Input: part model. Units: mm. Frame: model coordinates. Face numbers are marked on the shaded views. A direction names the side the tool comes from. Give positions to 0.01 mm unless a question says otherwise; leave off trailing zeros. Write each loop counter-clockwise with the first axis right and the second up, starting at its lowest first coordinate (ties: lowest second). Pieces come first, ordered by that corner, then holes. Notation, with made-up numbers: M -13,36 L 6,36 A22 ccw 6,47 Z; hole C -15.5,-38 d3. An arc over 180 degrees is marked long. Use CSV: the item, a comma, the result in double quotes. Start each with the question number.
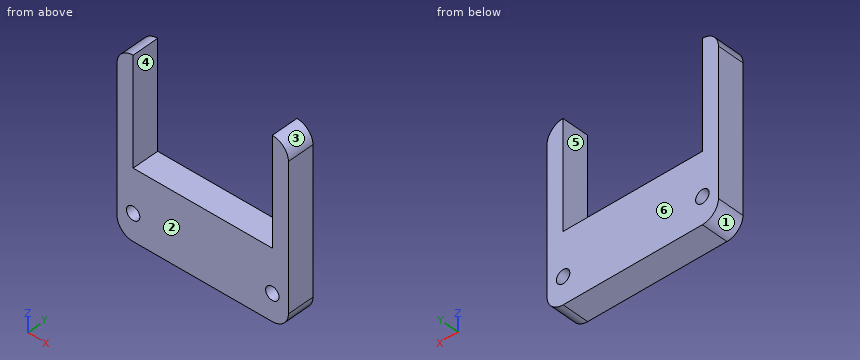
from build123d import *

# Parameters (mm, degrees)
SKETCH1_R           = 1.25
BOSS_EXTRUDE1_DEPTH = 5
FILLET1_R           = 3


with BuildPart() as part:
    # Sketch1 → Boss-Extrude1 (new body)
    with BuildSketch(Plane(origin=(0, 0, 0), x_dir=(1, 0, 0), z_dir=(0, 1, 0))):
        Polygon((29, 0), (32, 0), (32, 33), (0, 33), (0, 0), (3, 0), (3, 20), (29, 20), align=None)
        with Locations(Location((3, 28, 0), (0, 0, 270))):
            Circle(SKETCH1_R, mode=Mode.SUBTRACT)
        with Locations(Location((29, 28, 0), (0, 0, 270))):
            Circle(SKETCH1_R, mode=Mode.SUBTRACT)
    extrude(amount=BOSS_EXTRUDE1_DEPTH)

    # Fillet1
    fillet1_edges = [part.edges().sort_by_distance(p)[0] for p in [
        (0, 2.5, -33),
        (32, 2.5, -33),
        (32, 2.5, 0),
        (0, 2.5, 0),
    ]]
    fillet(fillet1_edges, radius=FILLET1_R - 0.0001)  # a hair under: the kernel refuses the full size


solid = part.part
Q1. Section D-D, the plane x = 22. Return the cut outline in (y, z).
Q2. Set-up query: the marked faces 5 and 6. Return all of +Z, -Z, +X, -X, +Y, -Y with unobstructed straight access to the full face (end or side cutting, diameter ignored); none if empty.
Q3. Section B-B, the plane z = -5. Return the cut outline in (x, y), and give its area (3 significant figures).
Q4. First-contact query: pin 1 Ø2 at (x, y) = (26.5, 4) entering from +Z. Flat tip, straight axial feed; report the tip coordinate or a pass-through.
Q5. Section C-C, the plane y = 4.15. Give the number of separate pieces and of enclosed holes in the cut face, and give its area (3 significant figures).
Q6. Section A-A, the plane z = -28. Return the cut outline in (x, y), and give its area (3 significant figures).
Q7. Material intervals for L1, parallel to X at y = 3.7, z = -28; L2, parallel to X at y = 0.8, z = -9.5; L3, parallel to Z at x = 22, y = 4.45, sorted ascending. Write a range as [from, to].
Q8. Pull-direction query (X, two-part tool) for the marked faces 1, 2, 3 and 4; classes: released by +X, released by -X, zero draft, split by the parting line, or undercut.
Check result:
1,outline,"M 0,-33 L 5,-33 L 5,-20 L 0,-20 Z"
2,face 5,"+Z, +Y, -Y"
2,face 6,"+Z, -Z, +X, -X, +Y"
3,outline,"M 0,0 L 3,0 L 3,5 L 0,5 Z; M 29,0 L 32,0 L 32,5 L 29,5 Z"
3,area,"30.0 mm²"
4,pin 1,"stops at z = -20"
5,separate pieces,"1"
5,enclosed holes,"2"
5,area,"518 mm²"
6,outline,"M 0,0 L 1.75,0 L 1.75,5 L 0,5 Z; M 4.25,0 L 27.75,0 L 27.75,5 L 4.25,5 Z; M 30.25,0 L 32,0 L 32,5 L 30.25,5 Z"
6,area,"135 mm²"
7,L1,"x = [0, 1.75], [4.25, 27.75], [30.25, 32]"
7,L2,"x = [0, 3], [29, 32]"
7,L3,"z = [-33, -20]"
8,face 1,"released by -X"
8,face 2,"zero draft"
8,face 3,"released by +X"
8,face 4,"undercut"
